Check sheet for the modelled part. Datum: model origin and axes. Units: mm. A direction names the side the tool comes from. Coordinates: 2 decimals unless noted, no trailing zeros. Write each loop counter-clockwise with the first axis right and the second up, starting at its lowest first coordinate (ties: lowest second). Pieces come first, ordered by that corner, then holes. Notation, with made-up numbers: M 65,-19.75 L 90,-19.75 A21 cw 90,6.25 Z; hole C 2.5,56.5 d8. An arc over 180 degrees is marked long. Answer as CSV lines item,"result". Start each with the question number.
Q1. Access from +Z, -Z, +X, -X, +Y, -Y to the whole of each face (thin tool, end or side, straight path). Record for faces 5 (the flat face through (-7, 37.701, 9)), 6 (the flat face through (-23.102, 12, 10)), 7 (the flat face through (16.898, 33, 10)).
Q2. Mould release check, pull along Z, two halves, no side actions. Record for faces 1 (the flat face through (-3, 17, 0)), 2 (the cylindrical face through (-26.841, 28.109, 16.983)), 3 (the flat face through (20, 29.597, 10)), 4 (the flat face through (20, 28, 19.981)): pulls with the +Z half, pulls with the -Z half, needs draft (parallel to the pull), parting line crosses it, or undercut.
Q3. Thickness scan on line 1 along X through (y, z) = (27.25, 15); line 2 along Y through (x, z) = (19, 8); line 3 along Y through (x, z) = (10, 5.75). Record the ranges inside material, lowest first. Write a range as from..to.
Q4. Sectioned sample at C-C, the plane z = 5.75. Count the separate pieces of the cut face and the enclosed holes in it, then the cut area to 3 significant figures.
Q5. Depth check by flat-ended pin: pin 1 Ø4 at (x, y) = (-20, 15.5) entering from -Z; pin 2 Ø1.5 at (x, y) = (19, 28) entering from +Z; pin 3 Ø8 at (y, z) = (13, 6) entering from -X; pin 4 Ø10 at (x, z) = (18.5, 12.5) entering from -Y. Enter the tip coordinate at first touch or a pass-through.
Q6. Sectioned sample at D-D, the plane x = 0.5. Record the cut outline in (y, z), then the cut area to 3 significant figures.
Q7. Sectioned sample at A-A, the plane z = 10. Record the cut outline in (x, y).
Q8. Sectioned sample at B-B, the plane y = 15. Record the cut outline in (x, z).
from build123d import *

# Parameters (mm, degrees)
SKETCH_1_W               = 40
SKETCH_1_H               = 39
EXTRUDE_1_DEPTH          = 20
SKETCH_3_W               = 20
SKETCH_3_H               = 3
EXTRUDE_2_DEPTH          = 8
SKETCH_6_W               = 20.033379722
SKETCH_6_H               = 3
EXTRUDE_4_DEPTH          = 8
CUT_EXTRUDE_1_DEPTH      = 38
CUT_EXTRUDE_1_DEPTH_BACK = 50
SKETCH_7_R               = 2
SKETCH_8_R               = 2
CUT_EXTRUDE_2_DEPTH      = 50
SKETCH_9_R               = 3
EXTRUDE_7_DEPTH          = 6
SKETCH_11_R              = 5.970559472
EXTRUDE_8_DEPTH          = 1.5
SKETCH_12_R              = 7.325621725
EXTRUDE_9_DEPTH          = 1
FILLET_3_R               = 1
FILLET_4_R               = 1
FILLET_5_R               = 1
FILLET_8_R               = 1
FILLET_9_R               = 1


with BuildPart() as part:
    # 草图1 → 凸台-拉伸1 (new body)
    with BuildSketch(Plane.XY):
        with Locations((-3.101604278, 17.200534759)):
            Rectangle(SKETCH_1_W, SKETCH_1_H)
    extrude(amount=EXTRUDE_1_DEPTH)

    # 草图3 → 凸台-拉伸2 (add)
    with BuildSketch(Plane(origin=(16.898395722, 0, 0), x_dir=(0, 0, -1), z_dir=(1, 0, 0))):
        with Locations((-9.980536854, 28.09692648)):
            Rectangle(SKETCH_3_W, SKETCH_3_H)
    extrude(amount=EXTRUDE_2_DEPTH)

    # 草图6 → 凸台-拉伸4 (add)
    with BuildSketch(Plane.ZY.offset(23.101604278)):
        with Locations((9.983310139, 28.130306202)):
            Rectangle(SKETCH_6_W, SKETCH_6_H)
    extrude(amount=EXTRUDE_4_DEPTH)

    # 草图7 → 切除-拉伸1 (cut, two sides: drawn at the far end of the back side and taken through both)
    with BuildSketch(Plane(origin=(0, 0, 0), x_dir=(1, 0, 0), z_dir=(0, 1, 0)).offset(-CUT_EXTRUDE_1_DEPTH_BACK)):
        with Locations(Location((-27.101604278, -15, 0), (0, 0, 180))):
            Circle(SKETCH_7_R)
        with Locations(Location((-27.101604278, -4.966620278, 0), (0, 0, 180))):
            Circle(SKETCH_7_R)
    extrude(amount=CUT_EXTRUDE_1_DEPTH + CUT_EXTRUDE_1_DEPTH_BACK, mode=Mode.SUBTRACT)

    # 草图8 → 切除-拉伸2 (cut)
    with BuildSketch(Plane(origin=(0, 29.59692648, 0), x_dir=(1, 0, 0), z_dir=(0, 1, 0))):
        with Locations(Location((20.898395722, -5, 0), (0, 0, 180))):
            Circle(SKETCH_8_R)
        with Locations(Location((20.898395722, -14.980536854, 0), (0, 0, 180))):
            Circle(SKETCH_8_R)
    extrude(amount=-CUT_EXTRUDE_2_DEPTH, mode=Mode.SUBTRACT)

    # 草图9 → 凸台-拉伸7 (add)
    with BuildSketch(Plane(origin=(0, 36.700534759, 0), x_dir=(1, 0, 0), z_dir=(0, 1, 0))):
        with Locations(Location((-13.101604278, -10, 0), (0, 0, 90))):
            Circle(SKETCH_9_R)
    extrude(amount=EXTRUDE_7_DEPTH)

    # 草图11 → 凸台-拉伸8 (add)
    with BuildSketch(Plane(origin=(0, 36.700534759, 0), x_dir=(1, 0, 0), z_dir=(0, 1, 0))):
        with Locations(Location((-13.101604278, -10, 0), (0, 0, 90))):
            Circle(SKETCH_11_R)
    extrude(amount=EXTRUDE_8_DEPTH)

    # 草图12 → 凸台-拉伸9 (add)
    with BuildSketch(Plane(origin=(0, 36.700534759, 0), x_dir=(1, 0, 0), z_dir=(0, 1, 0))):
        with Locations(Location((-13.101604278, -10, 0), (0, 0, 90))):
            Circle(SKETCH_12_R)
    extrude(amount=EXTRUDE_9_DEPTH)

    # 圆角3
    # the kernel refuses this fillet: 1 mm, written as the material it takes off along each edge
    with BuildSketch(Plane(origin=(15.898395722, 35.700534759, 19), x_dir=(0, 0, 1), z_dir=(0, 1, 0))) as fillet_3_piece_1_section:
        Polygon((0, 0), (FILLET_3_R, 0), (FILLET_3_R, FILLET_3_R), (0, FILLET_3_R), align=None)
    fillet_3_piece_1 = extrude(amount=FILLET_3_R, mode=Mode.PRIVATE)
    fillet_3_piece_1 = fillet_3_piece_1 - Plane(origin=(15.898395722, 35.700534759, 19), x_dir=(-0.7071067811865475, 0, -0.7071067811865475), z_dir=(0, 1, 0)) * Sphere(FILLET_3_R, mode=Mode.PRIVATE)
    add(fillet_3_piece_1, mode=Mode.SUBTRACT)
    with BuildSketch(Plane(origin=(16.898395722, 36.700534759, -2.5), x_dir=(-1, 0, 0), z_dir=(0, 0, 1))) as fillet_3_piece_2:
        with BuildLine():
            CenterArc((FILLET_3_R, FILLET_3_R), FILLET_3_R, 180, 90)
            Line((0, FILLET_3_R), (0, 0))
            Line((0, 0), (FILLET_3_R, 0))
        make_face()
    extrude(amount=21.5, mode=Mode.SUBTRACT)
    with BuildSketch(Plane(origin=(16.898395722, 35.700534759, 20), x_dir=(-1, 0, 0), z_dir=(0, -1, 0))) as fillet_3_piece_3_section:
        with BuildLine():
            CenterArc((FILLET_3_R, FILLET_3_R), FILLET_3_R, 180, 90)
            Line((0, FILLET_3_R), (0, 0))
            Line((0, 0), (FILLET_3_R, 0))
        make_face()
    fillet_3_piece_3 = extrude(amount=40.5, mode=Mode.PRIVATE)
    fillet_3_piece_3 = split(fillet_3_piece_3, bisect_by=Plane(origin=(16.437934638, 29.59692648, 20.00107683), z_dir=(0, 1, 0)), keep=Keep.TOP, mode=Mode.PRIVATE)
    fillet_3_piece_3 = split(fillet_3_piece_3, bisect_by=Plane(origin=(16.437934638, 32.648730619, 19.980536854), z_dir=(0, 0, 1)), keep=Keep.TOP, mode=Mode.PRIVATE)
    add(fillet_3_piece_3, mode=Mode.SUBTRACT)
    with BuildSketch(Plane(origin=(16.898395722, 35.700534759, 20), x_dir=(-1, 0, 0), z_dir=(0, -1, 0))) as fillet_3_piece_4_section:
        with BuildLine():
            CenterArc((FILLET_3_R, FILLET_3_R), FILLET_3_R, 180, 90)
            Line((0, FILLET_3_R), (0, 0))
            Line((0, 0), (FILLET_3_R, 0))
        make_face()
    fillet_3_piece_4 = extrude(amount=40.5, mode=Mode.PRIVATE)
    fillet_3_piece_4 = split(fillet_3_piece_4, bisect_by=Plane(origin=(16.712608884, 29.59692648, 19.734140611), z_dir=(0, 1, 0)), keep=Keep.TOP, mode=Mode.PRIVATE)
    fillet_3_piece_4 = split(fillet_3_piece_4, bisect_by=Plane(origin=(16.712608884, 32.648730619, 19.980536854), z_dir=(0, 0, -1)), keep=Keep.TOP, mode=Mode.PRIVATE)
    add(fillet_3_piece_4, mode=Mode.SUBTRACT)
    with BuildSketch(Plane(origin=(16.898395722, 35.700534759, 20), x_dir=(-1, 0, 0), z_dir=(0, -1, 0))) as fillet_3_piece_5_section:
        with BuildLine():
            CenterArc((FILLET_3_R, FILLET_3_R), FILLET_3_R, 180, 90)
            Line((0, FILLET_3_R), (0, 0))
            Line((0, 0), (FILLET_3_R, 0))
        make_face()
    fillet_3_piece_5 = extrude(amount=40.5, mode=Mode.PRIVATE)
    fillet_3_piece_5 = split(fillet_3_piece_5, bisect_by=Plane(origin=(16.437934638, 29.59692648, 20.00107683), z_dir=(0, -1, 0)), keep=Keep.TOP, mode=Mode.PRIVATE)
    fillet_3_piece_5 = split(fillet_3_piece_5, bisect_by=Plane(origin=(16.437934638, 28.09692648, 19.980536854), z_dir=(0, 0, 1)), keep=Keep.TOP, mode=Mode.PRIVATE)
    fillet_3_piece_5 = split(fillet_3_piece_5, bisect_by=Plane(origin=(16.437934638, 26.59692648, 20.00107683), z_dir=(0, 1, 0)), keep=Keep.TOP, mode=Mode.PRIVATE)
    add(fillet_3_piece_5, mode=Mode.SUBTRACT)
    with BuildSketch(Plane(origin=(16.898395722, 35.700534759, 20), x_dir=(-1, 0, 0), z_dir=(0, -1, 0))) as fillet_3_piece_6_section:
        with BuildLine():
            CenterArc((FILLET_3_R, FILLET_3_R), FILLET_3_R, 180, 90)
            Line((0, FILLET_3_R), (0, 0))
            Line((0, 0), (FILLET_3_R, 0))
        make_face()
    fillet_3_piece_6 = extrude(amount=40.5, mode=Mode.PRIVATE)
    fillet_3_piece_6 = split(fillet_3_piece_6, bisect_by=Plane(origin=(16.437934638, 10.898730619, 19.980536854), z_dir=(0, 0, 1)), keep=Keep.TOP, mode=Mode.PRIVATE)
    fillet_3_piece_6 = split(fillet_3_piece_6, bisect_by=Plane(origin=(16.437934638, 26.59692648, 20.00107683), z_dir=(0, -1, 0)), keep=Keep.TOP, mode=Mode.PRIVATE)
    add(fillet_3_piece_6, mode=Mode.SUBTRACT)
    with BuildSketch(Plane(origin=(16.898395722, 35.700534759, 20), x_dir=(-1, 0, 0), z_dir=(0, -1, 0))) as fillet_3_piece_7_section:
        with BuildLine():
            CenterArc((FILLET_3_R, FILLET_3_R), FILLET_3_R, 180, 90)
            Line((0, FILLET_3_R), (0, 0))
            Line((0, 0), (FILLET_3_R, 0))
        make_face()
    fillet_3_piece_7 = extrude(amount=40.5, mode=Mode.PRIVATE)
    fillet_3_piece_7 = split(fillet_3_piece_7, bisect_by=Plane(origin=(16.712608884, 10.898730619, 19.980536854), z_dir=(0, 0, -1)), keep=Keep.TOP, mode=Mode.PRIVATE)
    fillet_3_piece_7 = split(fillet_3_piece_7, bisect_by=Plane(origin=(16.712608884, 26.59692648, 19.734140611), z_dir=(0, -1, 0)), keep=Keep.TOP, mode=Mode.PRIVATE)
    add(fillet_3_piece_7, mode=Mode.SUBTRACT)
    with BuildSketch(Plane(origin=(-25.601604278, 36.700534759, 20), x_dir=(0, 0, -1), z_dir=(1, 0, 0))) as fillet_3_piece_8:
        with BuildLine():
            CenterArc((FILLET_3_R, -FILLET_3_R), FILLET_3_R, 90, 90)
            Line((0, -FILLET_3_R), (0, 0))
            Line((0, 0), (FILLET_3_R, 0))
        make_face()
    extrude(amount=41.5, mode=Mode.SUBTRACT)

    # 圆角4
    fillet_4_edges = [part.edges().sort_by_distance(p)[0] for p in [
        (-23.101604278, 12.16542048, 0),
        (-23.101604278, 12.16542048, 20),
        (-3.101604278, -2.299465241, 0),
        (-23.101604278, -2.299465241, 10),
        (-3.601604278, -2.299465241, 20),
        (16.898395722, -2.299465241, 9.5),
        (16.605502503, -2.299465241, 19.707106781),
    ]]
    fillet(fillet_4_edges, radius=FILLET_4_R)

    # 圆角5
    # the kernel refuses this fillet: 1 mm, written as the material it takes off along each edge
    with BuildSketch(Plane(origin=(15.898395722, -1.299465241, 1), x_dir=(1, 0, 0), z_dir=(0, 0, -1))) as fillet_5_piece_1_section:
        Polygon((0, 0), (FILLET_5_R * 1.02, 0), (FILLET_5_R * 1.02, FILLET_5_R * 1.02), (0, FILLET_5_R * 1.02), align=None)
    fillet_5_piece_1 = extrude(amount=FILLET_5_R * 1.02, mode=Mode.PRIVATE)
    fillet_5_piece_1 = fillet_5_piece_1 - Plane(origin=(15.898395722, -1.299465241, 1), x_dir=(-0.7071067811865476, 0.7071067811865475, 0), z_dir=(0, 0, -1)) * Sphere(FILLET_5_R, mode=Mode.PRIVATE)
    add(fillet_5_piece_1, mode=Mode.SUBTRACT)
    with BuildSketch(Plane(origin=(-22.101604278, 35.700534759, 1), x_dir=(-1, 0, 0), z_dir=(0, 0, -1))) as fillet_5_piece_2_section:
        Polygon((0, 0), (FILLET_5_R * 1.02, 0), (FILLET_5_R * 1.02, FILLET_5_R * 1.02), (0, FILLET_5_R * 1.02), align=None)
    fillet_5_piece_2 = extrude(amount=FILLET_5_R * 1.02, mode=Mode.PRIVATE)
    fillet_5_piece_2 = fillet_5_piece_2 - Plane(origin=(-22.101604278, 35.700534759, 1), x_dir=(0.7071067811865476, -0.7071067811865475, 0), z_dir=(0, 0, -1)) * Sphere(FILLET_5_R, mode=Mode.PRIVATE)
    add(fillet_5_piece_2, mode=Mode.SUBTRACT)
    with BuildSketch(Plane(origin=(16.898395722, 26.59692648, 0), x_dir=(-1, 0, 0), z_dir=(0, -1, 0))) as fillet_5_piece_3:
        with BuildLine():
            CenterArc((FILLET_5_R, -FILLET_5_R), FILLET_5_R, 90, 90)
            Line((0, -FILLET_5_R), (0, 0))
            Line((0, 0), (FILLET_5_R, 0))
        make_face()
    extrude(amount=27.89639172, mode=Mode.SUBTRACT)
    with BuildSketch(Plane(origin=(16.898395722, 35.700534759, 0), x_dir=(-1, 0, 0), z_dir=(0, -1, 0))) as fillet_5_piece_4:
        with BuildLine():
            CenterArc((FILLET_5_R, -FILLET_5_R), FILLET_5_R, 90, 90)
            Line((0, -FILLET_5_R), (0, 0))
            Line((0, 0), (FILLET_5_R, 0))
        make_face()
    extrude(amount=6.10360828, mode=Mode.SUBTRACT)
    with BuildSketch(Plane(origin=(-23.101604278, 29.630306202, 0), x_dir=(1, 0, 0), z_dir=(0, 1, 0)), Plane(origin=(-23.101604278, 29.630306202, 20), x_dir=(0, 0, -1), z_dir=(0, 1, 0))) as fillet_5_piece_5:
        with BuildLine():
            CenterArc((FILLET_5_R, -FILLET_5_R), FILLET_5_R, 90, 90)
            Line((0, -FILLET_5_R), (0, 0))
            Line((0, 0), (FILLET_5_R, 0))
        make_face()
    extrude(amount=6.070228558, mode=Mode.SUBTRACT)
    with BuildSketch(Plane(origin=(-22.101604278, 36.700534759, 0), x_dir=(0, -1, 0), z_dir=(1, 0, 0))) as fillet_5_piece_6:
        with BuildLine():
            CenterArc((FILLET_5_R, -FILLET_5_R), FILLET_5_R, 90, 90)
            Line((0, -FILLET_5_R), (0, 0))
            Line((0, 0), (FILLET_5_R, 0))
        make_face()
    extrude(amount=38, mode=Mode.SUBTRACT)
    with BuildSketch(Plane(origin=(-23.101604278, 36.700534759, 1), x_dir=(0, -1, 0), z_dir=(0, 0, 1))) as fillet_5_piece_7:
        with BuildLine():
            CenterArc((FILLET_5_R, FILLET_5_R), FILLET_5_R, 180, 90)
            Line((0, FILLET_5_R), (0, 0))
            Line((0, 0), (FILLET_5_R, 0))
        make_face()
    extrude(amount=18, mode=Mode.SUBTRACT)
    with BuildSketch(Plane(origin=(15.898395722, 35.700534759, 0), x_dir=(0, 1, 0), z_dir=(-1, 0, 0))) as fillet_5_piece_8:
        with BuildLine():
            CenterArc((1 - FILLET_5_R, -FILLET_5_R), FILLET_5_R, 0, 90)
            Line((1, -FILLET_5_R), (1, 0))
            Line((1, 0), (1 - FILLET_5_R, 0))
        make_face()
    revolve(axis=Axis((15.898395722, 35.700534759, 0), (0, 0, -1)), revolution_arc=90, mode=Mode.SUBTRACT)
    with BuildSketch(Plane(origin=(-23.101604278, 35.700534759, 19), x_dir=(0, 0, 1), z_dir=(0, -1, 0))) as fillet_5_piece_9:
        with BuildLine():
            CenterArc((1 - FILLET_5_R, -FILLET_5_R), FILLET_5_R, 0, 90)
            Line((1, -FILLET_5_R), (1, 0))
            Line((1, 0), (1 - FILLET_5_R, 0))
        make_face()
    revolve(axis=Axis((-23.101604278, 35.700534759, 19), (-1, 0, 0)), revolution_arc=90, mode=Mode.SUBTRACT)

    # 圆角8
    fillet_8_edges = [part.edges().sort_by_distance(p)[0] for p in [
        (24.898395722, 28.09692648, -0.019463146),
        (24.898395722, 28.09692648, 19.980536854),
    ]]
    fillet(fillet_8_edges, radius=FILLET_8_R)

    # 圆角9
    fillet_9_edges = [part.edges().sort_by_distance(p)[0] for p in [
        (-31.101604278, 28.130306202, 20),
        (-31.101604278, 28.130306202, -0.033379722),
    ]]
    fillet(fillet_9_edges, radius=FILLET_9_R)


solid = part.part
Output:
1,face 5,"+Y"
1,face 6,"+Z, -Z, -X, -Y"
1,face 7,"+Z, -Z, +X, +Y"
2,face 1,"pulls with the -Z half"
2,face 2,"undercut"
2,face 3,"needs draft"
2,face 4,"pulls with the +Z half"
3,line 1,"x = -31.1..-29.1, -25.1..18.9, 22.9..24.9"
3,line 2,"y = 26.6..29.6"
3,line 3,"y = -2.3..36.7"
4,separate pieces,"3"
4,enclosed holes,"0"
4,area,"1,600 mm^2"
5,pin 1,"stops at z = 0"
5,pin 2,"stops at z = 19.98"
5,pin 3,"stops at x = -23.1"
5,pin 4,"stops at y = -2.3"
6,outline,"M -2.3,1 A1 ccw -1.3,0 L 35.7,0 A1 ccw 36.7,1 L 36.7,19 A1 ccw 35.7,20 L -1.3,20 A1 ccw -2.3,19 Z"
6,area,"779 mm^2"
7,outline,"M -31.1,26.63 L -23.1,26.63 L -23.1,-1.3 A1 ccw -22.1,-2.3 L 15.9,-2.3 A1 ccw 16.9,-1.3 L 16.9,26.6 L 24.9,26.6 L 24.9,29.6 L 16.9,29.6 L 16.9,35.7 A1 ccw 15.9,36.7 L -5.78,36.7 L -5.78,37.7 L -7.13,37.7 L -7.13,38.2 L -10.1,38.2 L -10.1,42.7 L -16.1,42.7 L -16.1,38.2 L -19.07,38.2 L -19.07,37.7 L -20.43,37.7 L -20.43,36.7 L -22.1,36.7 A1 ccw -23.1,35.7 L -23.1,29.63 L -31.1,29.63 Z"
8,outline,"M -23.1,1 A1 ccw -22.1,0 L 15.9,0 A1 ccw 16.9,1 L 16.9,19 A1 ccw 15.9,20 L -22.1,20 A1 ccw -23.1,19 Z"
